Autodesk Fusion 360 part; units mm, degrees
sketch "Sketch1" plane through (0, 0, 0) normal (0, 0, 1) x (1, 0, 0)
  circle A0 centre (0, 0) radius 10
  circle A1 centre (0, 0) radius 12.5
  line L0 (0, 0) -> (135, 0) construction
  circle A2 centre (135, 0) radius 10
  circle A3 centre (135, 0) radius 12.5
  line L1 (0, 12.5) -> (135, 12.5)
  line L2 (0, -12.5) -> (135, -12.5)
  circle A4 centre (20, 0) radius 2.5
  circle A5 centre (55, 0) radius 2.5
  circle A6 centre (0, 0) radius 1.5
  circle A7 centre (135, 0) radius 1.5
  dimension "d1" = 20
  dimension "d2" = 25
  dimension "d3" = 20
  dimension "d5" = 135
  dimension "d6" = 5
  dimension "d7" = 5
  dimension "d8" = 35
  dimension "d9" = 20
  dimension "d16" = 3
  dimension "d17" = 3
extrude "Extrude1" add sketch "Sketch1" along normal blind 10 contours A1 A3 L1 L2 makes body 1
extrude "Extrude2" add sketch "Sketch1" along normal blind 5 separate body contours A0 | A2 | A6 | A7 makes body 2 at (9.9876, -0.4985, 3.3333) makes body 3 at (131.9968, 2.3092, 0)
extrude "Extrude3" add sketch "Sketch1" along normal blind 20 contours A1 | A3 bodies 1 2 3
extrude "Extrude4" cut sketch "Sketch1" along normal through all contours A6 | A7 bodies 1
chamfer "Chamfer1" distance 1 angle 45 1 faces at (108.6406, -4.5163, 0) on bodies 1
chamfer "Chamfer2" distance 1 angle 45 2 edges at (67.5, 12.5, 10) (67.5, -12.5, 10) on bodies 1
Check sheet for the modelled part. Datum: model origin and axes. Units: mm. A direction names the side the tool comes from. Round coordinates to 2 decimals unless told otherwise and drop trailing zeros. Order: outer loops, then holes, each group sorted by start corner. A loop starts at its lowest first (then second) coordinate and runs counter-clockwise, first axis right, second up.
1) Mould release check, pull along Y, two halves, no side actions. Record for faces 3 (the cylindrical face through (133.5, -0.07, 2.97)), 4 (the flat face through (66, 0, 0)), 5 (the conical face through (146.671, -0.257, 0.174)): +Y half, -Y half, draft (parallel to the pull), parting line (faces both ways), or undercut.
2) Section check A-A (x = 55). Record the boundary of the cut face in (y, z), and give its area (3 significant figures).
3) Go/stop test with flat-tipped pins: pin 1 Ø6 at (x, y) = (77, -1) entering from -Z; pin 2 Ø1.5 at (y, z) = (-2, 17.5) entering from -X; pin 3 Ø2.5 at (x, y) = (0, 0) entering from -Z; pin 4 Ø2 at (y, z) = (4.5, 9) entering from +X. Record where each tip stops, or that it passes through.
4) Scan lines: line 1 (X direction, y = 5, z = 12.25); line 2 (Y direction, x = 135, z = 9.25); line 3 (X direction, y = 8.5, z = 8.5). Record each from-to range of solid material in increasing order.
5) Tool access check on faces 1 (the cylindrical face through (57.31, 0.96, 5.44)), 2 (the cylindrical face through (144.237, 3.83, 12.395)). Record the directions out of +Z, -Z, +X, -X, +Y, -Y that give a thin tool (end or side, any length) a straight path to the whole face; none if there is none.
6) Section check B-B (y = 0). Give the number of separate pieces and of enclosed holes in the cut face, and give its area (4 significant figures).
7) Section check C-C (x = 84.5). Record the boundary of the cut face in (y, z).
Result:
1. face 3: undercut
1. face 4: draft
1. face 5: parting line
2. outline: (-12.5, 1) - (-11.5, 0) - (-3.5, 0) - (-2.5, 1) - (-2.5, 10) - (-11.5, 10) - (-12.5, 9) - close; (2.5, 1) - (3.5, 0) - (11.5, 0) - (12.5, 1) - (12.5, 9) - (11.5, 10) - (2.5, 10) - close
2. area: 197 mm2
3. pin 1: stops at z = 0
3. pin 2: stops at x = -12.44
3. pin 3: passes through
3. pin 4: stops at x = 147
4. line 1: x = -11.46 to -8.66, 8.66 to 11.46, 123.54 to 126.34, 143.66 to 146.46
4. line 2: y = -12.5 to -10, 10 to 12.5
4. line 3: x = -9.17 to -5.27, 5.27 to 129.73, 140.27 to 144.17
5. face 1: +Z, -Z
5. face 2: +Z
6. separate pieces: 5
6. enclosed holes: 0
6. area: 1,365 mm2
7. outline: (-12.5, 1) - (-11.5, 0) - (11.5, 0) - (12.5, 1) - (12.5, 9) - (11.5, 10) - (-11.5, 10) - (-12.5, 9) - close
